Here's how the part is built. I have some questions about the finished solid (model axes, mm). Give positions to 0.01 mm unless a question says otherwise; leave off trailing zeros. Write each loop counter-clockwise with the first axis right and the second up, starting at its lowest first coordinate (ties: lowest second). Pieces come first, ordered by that corner, then holes. Notation, with made-up numbers: (65, 4.5) -> (109, 4.5) arc R16 cw to (109, 27.5) -> close; hole circle Ø11 at (63, 77). An arc over 180 degrees is marked (long way). Return JSON: item names as keys, results as strings.
from build123d import *

# Parameters (mm, degrees)
CYLINDER014005822_R     = 51
CYLINDER014005822_DEPTH = 12
BOX001_W                = 10
BOX001_H                = 12
BOX001_DEPTH            = 40


with BuildPart() as obj1:
    # Cylinder014005822 → Cylinder014005822 (new body)
    with BuildSketch(Plane.XZ.offset(-51.5)):
        Circle(CYLINDER014005822_R)
    extrude(amount=CYLINDER014005822_DEPTH)


with BuildPart() as obj2:
    # Box001 → Box001 (new body)
    with BuildSketch(Plane(origin=(43, 39.5, -20), x_dir=(1, 0, 0), z_dir=(0, 0, 1))):
        with Locations((5, 6)):
            Rectangle(BOX001_W, BOX001_H)
    extrude(amount=BOX001_DEPTH)

    # Cut009003003003: cut obj1
    add(obj1.part, mode=Mode.SUBTRACT)


solid = obj2.part
1. Suppose I cut it at B-B, the plane y = 45.5. List the corners of the cut face in (x, z) for me, and give its area (3 significant figures).
Taken from the geometry:
{"outline": "(46.91, -20) -> (53, -20) -> (53, 20) -> (46.91, 20) arc R51 cw to start", "area": "134 mm²"}
2. If I drill on line 1 (X direction, y = 42.25, z = 2.5); line 2 (X direction, y = 44, z = -5.5), over which ranges is the centre line in solid material (lowest first)? Write a range as [from, to].
Taken from the geometry:
{"line 1": "x = [50.94, 53]", "line 2": "x = [50.7, 53]"}
3. Suppose I cut it at C-C, the plane x = 49.5. List the corners of the cut face in (y, z) for me, and give its area (3 significant figures).
Taken from the geometry:
{"outline": "(39.5, -20) -> (51.5, -20) -> (51.5, -12.28) -> (39.5, -12.28) -> close; (39.5, 12.28) -> (51.5, 12.28) -> (51.5, 20) -> (39.5, 20) -> close", "area": "185 mm²"}
4. Suppose I cut it at A-A, the plane x = 48. List the corners of the cut face in (y, z) for me, and give its area (3 significant figures).
Taken from the geometry:
{"outline": "(39.5, -20) -> (51.5, -20) -> (51.5, -17.23) -> (39.5, -17.23) -> close; (39.5, 17.23) -> (51.5, 17.23) -> (51.5, 20) -> (39.5, 20) -> close", "area": "66.4 mm²"}
5. Suppose I cut it at D-D, the plane z = 16.5. List the corners of the cut face in (x, y) for me, and give its area (3 significant figures).
Taken from the geometry:
{"outline": "(48.26, 39.5) -> (53, 39.5) -> (53, 51.5) -> (48.26, 51.5) -> close", "area": "56.9 mm²"}
